Check sheet for the modelled part. Datum: model origin and axes. Units: mm. Face numbers are marked on the shaded views. A direction names the side the tool comes from. Give positions to 0.01 mm unless a question says otherwise; leave off trailing zeros. Answer in a Markdown table with one row per item. Add a question column.
(1) Draft check along Z on the marked faces 3, 4 and 5. Enter one of: released by +Z, released by -Z, zero draft, split by the parting line, or undercut.
(2) Go/stop test with flat-tipped pins: P1, Ø6, axis at x = 3.5, y = 1, coming from the -Z side; P2, Ø3, axis at x = 7, z = -6.5, coming from the +Y side; P3, Ø2, axis at x = 20, y = -5, coming from the -Z side; P4, Ø4, axis at y = 3.5, z = -0.5, coming from the +X side. Record where each tip stops, or that it passes through.
(3) Sectioned sample at A-A on y = 0.5. State how many separate pieces and enclosed holes the cut face has, then the cut area to 3 significant figures.
(4) Thickness scan on L1, parallel to Z at x = 21.75, y = 1.25; L2, parallel to X at y = -0.25, z = -6.25; L3, parallel to Z at x = 17.25, y = -1. Record the ranges inside material, lowest first.
(5) Set-up check for the marked faces 1 and 2: record each of +Z, -Z, +X, -X, +Y, -Y from which the full face is reachable in a straight line by a thin tool's end or side.
from build123d import *

# Parameters (mm, degrees)
BOSS_EXTRUDE1_DEPTH = 26
SKETCH3_R           = 0.8
CUT_EXTRUDE1_DEPTH  = 7


with BuildPart() as part:
    # Sketch1 → Boss-Extrude1 (new body)
    with BuildSketch(Plane(origin=(0, 0, 0), x_dir=(0, 0, -1), z_dir=(1, 0, 0))):
        with BuildLine():
            Line((3.5, 3.0625), (5.205065915, 6.046365351))
            Line((5.205065915, 6.046365351), (11.28276791, 2.573392782))
            Line((11.28276791, 2.573392782), (9.577701995, -0.410472568))
            add(Edge.make_bspline(
                [(-6.949747468, -3.949747468), (-6.685368266, -4.214126671), (-6.147554271, -4.708312104), (-4.8590745, -5.674523534), (-2.826984501, -6.712797376), (0.295880791, -7.18416331), (3.330320935, -6.524197206), (5.630020015, -5.201123324), (7.839744032, -3.168086519), (8.912819335, -1.574017223), (9.577701995, -0.410472568)],
                knots=[0.075491359, 0.075491359, 0.075491359, 0.075491359, 0.129884041, 0.184276723, 0.293062086, 0.401847449, 0.510632813, 0.619418176, 0.72820354, 0.945774267, 0.945774267, 0.945774267, 0.945774267], degree=3))
            Line((-6.949747468, -3.949747468), (-8.196862299, -2.702632638))
            Line((-8.196862299, -2.702632638), (-3.24711483, 2.24711483))
            Line((-3.24711483, 2.24711483), (-2, 1))
            add(Edge.make_bspline(
                [(-2, 1), (0.75, -1.75), (3.5, 3.0625)],
                knots=[0.075491359, 0.075491359, 0.075491359, 0.945774267, 0.945774267, 0.945774267], degree=2))
        make_face()
    extrude(amount=BOSS_EXTRUDE1_DEPTH)

    # Sketch3 → Cut-Extrude1 (cut)
    with BuildSketch(Plane(origin=(0, 7.641933234, -2.41282212), x_dir=(1, 0, 0), z_dir=(0, 0.868243142, -0.496138938))):
        with Locations((4, 6.715969882)):
            Circle(SKETCH3_R)
        with Locations((22, 6.715969882)):
            Circle(SKETCH3_R)
    extrude(amount=-CUT_EXTRUDE1_DEPTH, mode=Mode.SUBTRACT)


solid = part.part
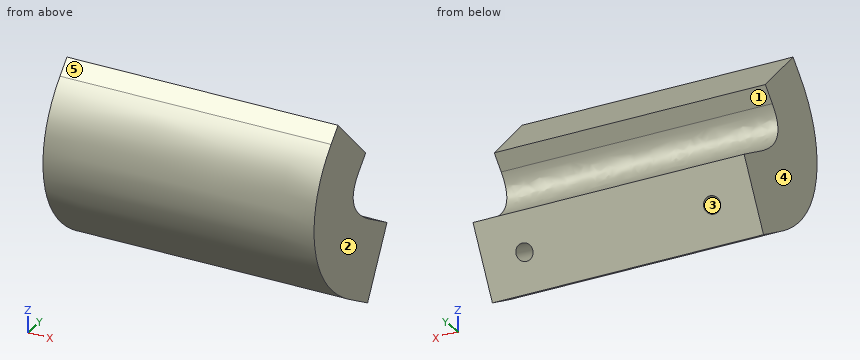
Reply:
| question | item | result |
|---|---|---|
| 1 | face 3 | undercut |
| 1 | face 4 | zero draft |
| 1 | face 5 | released by +Z |
| 2 | P1 | z = -11.28 |
| 2 | P2 | y = 6.05 |
| 2 | P3 | z = -6.9 |
| 2 | P4 | through |
| 3 | separate pieces | 2 |
| 3 | enclosed holes | 2 |
| 3 | area | 314 mm^2 |
| 4 | L1 | -10.53 to -7.37, -5.62 to -2.24, 2.25 to 4.24 |
| 4 | L2 | 0 to 3.4, 4.6 to 21.4, 22.6 to 26 |
| 4 | L3 | -9.23 to 6.49 |
| 5 | face 1 | +X, -X, +Y |
| 5 | face 2 | +Z, -Z, +X, +Y, -Y |
